Read the model definition and answer for the solid it produces. Units are mm, in the model's axes. A direction names the side the tool comes from. Give positions to 0.01 mm unless a question says otherwise; leave off trailing zeros. Write each loop counter-clockwise with the first axis right and the second up, starting at its lowest first coordinate (ties: lowest second). Pieces come first, ordered by that corner, then holes. Notation, with made-up numbers: M 59.25,-12.75 L 81.25,-12.75 A26 cw 81.25,3.25 Z; hole C -5,73.25 d5. An arc over 180 degrees is marked long. Put each result on its own line as item: value.
Autodesk Inventor part; units mm, degrees
ref_plane "YZ Plane" through (0, 0, 0) normal (1, 0, 0) x (0, 1, 0)
ref_plane "XZ Plane" through (0, 0, 0) normal (0, 1, 0) x (-1, 0, 0)
ref_plane "XY Plane" through (0, 0, 0) normal (0, 0, 1) x (1, 0, 0)
sketch "Sketch1" plane through (0, 0, 0) normal (0, 0, 1) x (1, 0, 0)
  line L0 (0, 0) -> (0, -100)
  line L1 (0, -100) -> (30, -100)
  line L2 (30, -100) -> (30, -96)
  line L3 (30, -96) -> (4, -96)
  line L4 (4, -96) -> (4, 0)
  line L5 (4, 0) -> (0, 0)
  dimension "d0" = 100
  dimension "d1" = 30
  dimension "d2" = 4
  dimension "d3" = 26
extrude "Extrusion1" add sketch "Sketch1" along normal blind 42
sketch "Sketch2" plane through (4, -96, 0) normal (1, 0, 0) x (0, 0, -1)
  line L0 (-42, 96) -> (-42, -4)
  line L1 (0, 96) -> (0, -4)
  line L2 (-42, 96) -> (0, 96)
  line L3 (0, 96) -> (0, 0)
  line L4 (0, 0) -> (-42, 0)
  line L5 (-42, 0) -> (-42, 96)
  circle A0 centre (-36.5, 90.5) radius 1.75
  circle A1 centre (-5.5, 90.5) radius 1.75
  circle A2 centre (-36.5, 59.5) radius 1.75
  circle A3 centre (-5.5, 59.5) radius 1.75
  circle A4 centre (-21, 75) radius 12
  dimension "d6" = 96
  dimension "d7" = 3.5
  dimension "d8" = 5.5
  dimension "d9" = 5.5
  dimension "d10" = 3.5
  dimension "d11" = 5.5
  dimension "d12" = 5.5
  dimension "d14" = 3.5
  dimension "d15" = 3.5
  dimension "d16" = 31
  dimension "d17" = 31
  dimension "d18" = 5.5
  dimension "d19" = 5.5
  dimension "d20" = 24
  dimension "d21" = 21
  dimension "d22" = 15.5
extrude "Extrusion2" cut sketch "Sketch2" against normal blind 4 contours A0 | A1 | A2 | A3 | A4
sketch "Sketch3" plane through (4, -96, 0) normal (0, 1, 0) x (1, 0, 0)
  line L0 (-4, 0) -> (-4, -42)
  line L1 (26, 0) -> (26, -42)
  line L2 (-4, 0) -> (26, 0)
  line L3 (26, 0) -> (26, -42)
  line L4 (26, -42) -> (-4, -42)
  line L5 (-4, -42) -> (-4, 0)
  circle A0 centre (21, -5) radius 1.75
  circle A1 centre (21, -37) radius 1.75
  circle A2 centre (8, -21) radius 1.75
  dimension "d25" = 3.5
  dimension "d26" = 3.5
  dimension "d27" = 3.5
  dimension "d28" = 5
  dimension "d29" = 5
  dimension "d30" = 5
  dimension "d31" = 5
  dimension "d32" = 12
  dimension "d33" = 21
extrude "Extrusion3" cut sketch "Sketch3" against normal blind 4 contours A0 | A1 | A2
fillet "Fillet1" radius 3 1 edges at (4, -96, 21)
properties part number "Suporte Esquerdo"
(1) Straight lines are drawn through the part: line 1 along Z through (x, y) = (25, -97); line 2 along Y through (x, z) = (2.7, 5.5); line 3 along Z through (x, y) = (12, -98.5). For each, find the intervals that lie inside material, in ascending order. Write a range as from..to.
Result:
line 1: z = 0..3.25, 6.75..35.25, 38.75..42
line 2: y = -100..-38.25, -34.75..-7.25, -3.75..0
line 3: z = 0..19.25, 22.75..42
(2) Given pin 1 Ø3 at (y, z) = (-36.5, 5.5) entering from -X; pin 2 Ø5.5 at (x, z) = (25, 37) entering from +Y; pin 3 Ø21 at (y, z) = (-69.5, 28) entering from +X, each flat-ended and moving along its own axis, determine where each tip first touches the part or whether it passes through.
Result:
pin 1: passes through
pin 2: stops at y = -96
pin 3: stops at x = 4
(3) Section B-B on x = 25 is taken. Determine the outline of the cut face in (y, z).
Result:
outline: M -100,0 L -96,0 L -96,3.25 L -100,3.25 Z; M -100,6.75 L -96,6.75 L -96,35.25 L -100,35.25 Z; M -100,38.75 L -96,38.75 L -96,42 L -100,42 Z
(4) Section C-C on y = -5.5 is taken. Determine the outline of the cut face in (x, z), and give its area (3 significant figures).
Result:
outline: M 0,0 L 4,0 L 4,3.75 L 0,3.75 Z; M 0,7.25 L 4,7.25 L 4,34.75 L 0,34.75 Z; M 0,38.25 L 4,38.25 L 4,42 L 0,42 Z
area: 140 mm²
(5) Section D-D on z = 10.5 is taken. Determine the outline of the cut face in (x, y).
Result:
outline: M 0,-100 L 30,-100 L 30,-96 L 7,-96 A3 cw 4,-93 L 4,-26.81 L 0,-26.81 Z; M 0,-15.19 L 4,-15.19 L 4,0 L 0,0 Z
(6) Which of the six approach directions +Z, -Z, +X, -X, +Y, -Y give full straight-line access (tool end or side, diameter ignored) to faces 1 (the face through (19, -96, 21)), 2 (the face through (23.25, -97.97, 4.92))?
Result:
face 1: +Z, -Z, +X, +Y
face 2: +Y, -Y
(7) For a pull along Y with two mould halves and no side action, classify faces 3 (the face through (2.03, -10.88, 14.55)), 4 (the face through (11.772, -97.972, 19.265)), 5 (the face through (2.028, -6.17, 34.883)), 6 (the face through (4.86, -95.1, 21.29)) as +Y half, -Y half, draft (parallel to the pull), parting line (faces both ways), or undercut.
Result:
face 3: undercut
face 4: draft
face 5: undercut
face 6: +Y half
(8) Section A-A on z = 21 is taken. Determine the outline of the cut face in (x, y).
Result:
outline: M 0,-100 L 10.25,-100 L 10.25,-96 L 7,-96 A3 cw 4,-93 L 4,-33 L 0,-33 Z; M 0,-9 L 4,-9 L 4,0 L 0,0 Z; M 13.75,-100 L 30,-100 L 30,-96 L 13.75,-96 Z
